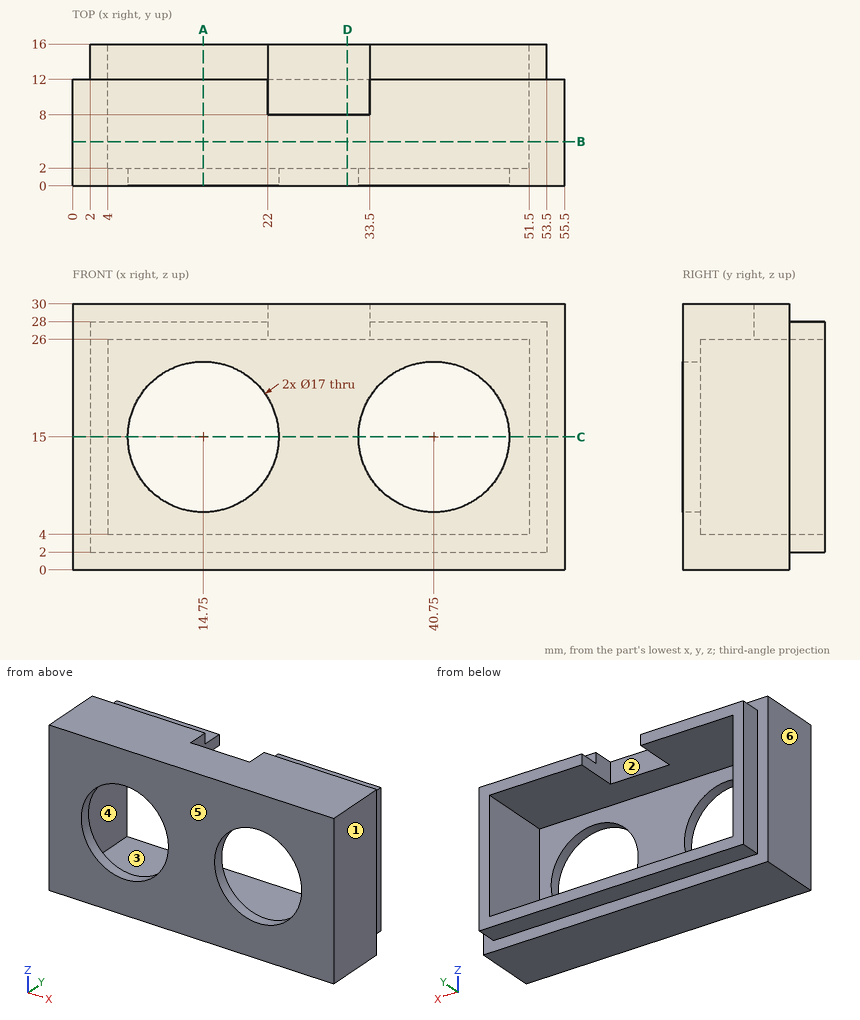
Can you work these out from the drawing? Everything is in mm from the part's minimum corner. A direction names the side the tool comes from. Round coordinates to 2 decimals unless told otherwise and drop trailing zeros. Loops run counter-clockwise (first coordinate to the right, second up) from the corner with the lowest first, then second, coordinate; pieces in that order, holes last. Notation, with made-up numbers: (72, -37.5) - (108, -37.5) arc R8 ccw to (108, -27.5) - close; hole circle Ø4 at (72.25, 7.25). An arc over 180 degrees is marked (long way). Answer in a Markdown table with one row per item. Add a question column.
Q1. I want a section at C-C on z = 15. List the corners of the cut face in (x, y) for me.
Q2. I need wall thicknesses on L1, parallel to X at y = 0.5, z = 15; L2, parallel to Z at x = 41.5, y = 10.5; L3, parallel to X at y = 14.5, z = 7.75. Which ranges of each line are inside material? Lowest first, please.
Q3. We'd pull the mould along X, two halves only. Please class the marked faces 4, 5 and 6: pulls with the +X half, pulls with the -X half, needs draft (parallel to the pull), parting line crosses it, or undercut.
Q4. I want a section at A-A on x = 14.75. List the corners of the cut face in (y, z) for me, and give its area (3 significant figures).
Q5. Which directions (+Z, -Z, +X, -X, +Y, -Y) give clear straight access to the entire face, cutting with the end or side of a thin tool? Please do the marked faces 1, 2 and 3.
Q6. I want a section at B-B on y = 5. List the corners of the cut face in (x, z) for me.
Q7. For pin 1 Ø5 at (x, z) = (38, 11.5) entering from +Y; pin 2 Ø4.5 at (y, z) = (15, 20) entering from +X; pin 3 Ø1 at (y, z) = (14, 16) entering from -X; pin 4 Ø1.2 at (x, y) = (41.5, 14) entering from +Z, each with a flat end and sliding along its axis, tell me the tip position at first contact or that it passes through.
Q8. I want a section at D-D on x = 31. List the corners of the cut face in (y, z) for me, and give its area (3 significant figures).
A:
| question | item | result |
|---|---|---|
| 1 | outline | (0, 0) - (6.25, 0) - (6.25, 2) - (4, 2) - (4, 16) - (2, 16) - (2, 12) - (0, 12) - close; (23.25, 0) - (32.25, 0) - (32.25, 2) - (23.25, 2) - close; (49.25, 0) - (55.5, 0) - (55.5, 12) - (53.5, 12) - (53.5, 16) - (51.5, 16) - (51.5, 2) - (49.25, 2) - close |
| 2 | L1 | 0 to 6.25, 23.25 to 32.25, 49.25 to 55.5 |
| 2 | L2 | 0 to 4, 26 to 30 |
| 2 | L3 | 2 to 4, 51.5 to 53.5 |
| 3 | face 4 | undercut |
| 3 | face 5 | needs draft |
| 3 | face 6 | pulls with the -X half |
| 4 | outline | (0, 0) - (12, 0) - (12, 2) - (16, 2) - (16, 4) - (2, 4) - (2, 6.5) - (0, 6.5) - close; (0, 23.5) - (2, 23.5) - (2, 26) - (16, 26) - (16, 28) - (12, 28) - (12, 30) - (0, 30) - close |
| 4 | area | 122 mm^2 |
| 5 | face 1 | +Z, -Z, +X, +Y, -Y |
| 5 | face 2 | +Z, +Y |
| 5 | face 3 | +Y |
| 6 | outline | (0, 0) - (55.5, 0) - (55.5, 30) - (0, 30) - close; hole (4, 4) - (51.5, 4) - (51.5, 26) - (4, 26) - close |
| 7 | pin 1 | through |
| 7 | pin 2 | x = 53.5 |
| 7 | pin 3 | x = 2 |
| 7 | pin 4 | z = 28 |
| 8 | outline | (0, 0) - (12, 0) - (12, 2) - (16, 2) - (16, 4) - (2, 4) - (2, 26) - (8, 26) - (8, 30) - (0, 30) - close |
| 8 | area | 132 mm^2 |
